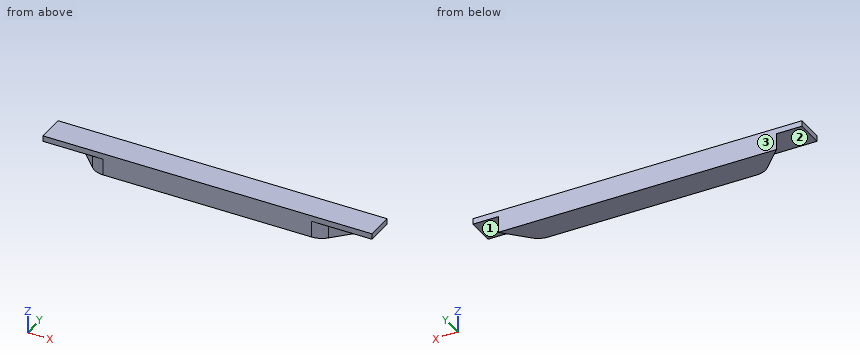
from build123d import *

# Parameters (mm, degrees)
Y_KSEKLIK_EKSTR_ZYON1_DEPTH = 2.6
IZIM2_W                     = 52
IZIM2_H                     = 4.388233566
Y_KSEKLIK_EKSTR_ZYON3_DEPTH = 0.9


with BuildPart() as part:
    # Çizim1 → Yükseklik-Ekstrüzyon1 (new body)
    with BuildSketch(Plane.XY):
        with BuildLine():
            Line((22, 4.388233566), (18.634136343, 0.912893359))
            ThreePointArc((18.634136343, 0.912893359), (17.649333458, 0.237635078), (16.479145422, 0))
            Line((16.479145422, 0), (-16.479145422, 0))
            ThreePointArc((-16.479145422, 0), (-17.649333458, 0.237635078), (-18.634136343, 0.912893359))
            Line((-18.634136343, 0.912893359), (-22, 4.388233566))
            Line((-22, 4.388233566), (22, 4.388233566))
        make_face()
    extrude(amount=Y_KSEKLIK_EKSTR_ZYON1_DEPTH)

    # Çizim2 → Yükseklik-Ekstrüzyon3 (add)
    with BuildSketch(Plane.XY.offset(2.6)):
        with Locations((0, 2.194116783)):
            Rectangle(IZIM2_W, IZIM2_H)
    extrude(amount=Y_KSEKLIK_EKSTR_ZYON3_DEPTH)


solid = part.part
Design review of the part built by this model. Coordinates are the model's own, in mm. Face numbers are marked on the shaded views. A direction names the side the tool comes from. Give positions to 0.01 mm unless a question says otherwise; leave off trailing zeros. Loops run counter-clockwise (first coordinate to the right, second up) from the corner with the lowest first, then second, coordinate; pieces in that order, holes last. Notation, with made-up numbers: M -8.75,14.25 L 17.25,14.25 A13 cw 17.25,25.25 Z; hole C 10,16.5 d5. An arc over 180 degrees is marked long. Answer as a JSON object with one key per item and string values.
Item 1: We need section D-D (y = 3.3). State the section outline as (x, z) points, and give its area (3 significant figures).
Output values:
{"outline": "M -26,2.6 L -20.95,2.6 L -20.95,0 L 20.95,0 L 20.95,2.6 L 26,2.6 L 26,3.5 L -26,3.5 Z", "area": "156 mm2"}
Item 2: We need section C-C (x = -21.5). State the section outline as (y, z) points, and give its area (3 significant figures).
Output values:
{"outline": "M 0,2.6 L 3.87,2.6 L 3.87,0 L 4.39,0 L 4.39,3.5 L 0,3.5 Z", "area": "5.29 mm2"}
Item 3: For P1, Ø1.3, axis at x = 23, y = 1.5, coming from the -Z side, flat-tipped, find the tip position at first contact; note if it passes through.
Output values:
{"P1": "stops at z = 2.6"}
Item 4: Wall thickness on line 1 along Z through (x, y) = (19.5, 0.6); line 2 along X through (y, z) = (2.3, 1.5); line 3 along Y through (x, z) = (17, 1.5): over which ranges is each line inside the solid? List them lowest first.
Output values:
{"line 1": "z = 2.6 to 3.5", "line 2": "x = -19.98 to 19.98", "line 3": "y = 0.05 to 4.39"}
Item 5: We need section B-B (y = 1.35). State the section outline as (x, z) points, and give its area (3 significant figures).
Output values:
{"outline": "M -26,2.6 L -19.06,2.6 L -19.06,0 L 19.06,0 L 19.06,2.6 L 26,2.6 L 26,3.5 L -26,3.5 Z", "area": "146 mm2"}
Item 6: Machinability: for the marked faces 1, 2 and 3, which of the approach directions +Z, -Z, +X, -X, +Y, -Y give a long, thin tool a straight path to every point of the face, cutting with its end or side? Answer none if there is none.
Output values:
{"face 1": "-Z, +X, -Y", "face 2": "-Z, -X, -Y", "face 3": "+Z, -Z, +X, -X, +Y"}
Item 7: We need section A-A (z = 0.85). State the section outline as (x, y) points.
Output values:
{"outline": "M -22,4.39 L -18.63,0.91 A3 ccw -16.48,0 L 16.48,0 A3 ccw 18.63,0.91 L 22,4.39 Z"}
